Work out the finished part from the listing and answer in its coordinate system (mm). Face numbers are marked on the shaded views. A direction names the side the tool comes from. Coordinates: 2 decimals unless noted, no trailing zeros. Order: outer loops, then holes, each group sorted by start corner. A loop starts at its lowest first (then second) coordinate and runs counter-clockwise, first axis right, second up. Notation, with made-up numbers: M 29.25,-4.75 L 51.25,-4.75 A23 ccw 51.25,15.25 Z; hole C 75,0.5 d8. An arc over 180 degrees is marked long. Use a Markdown table: item, result.
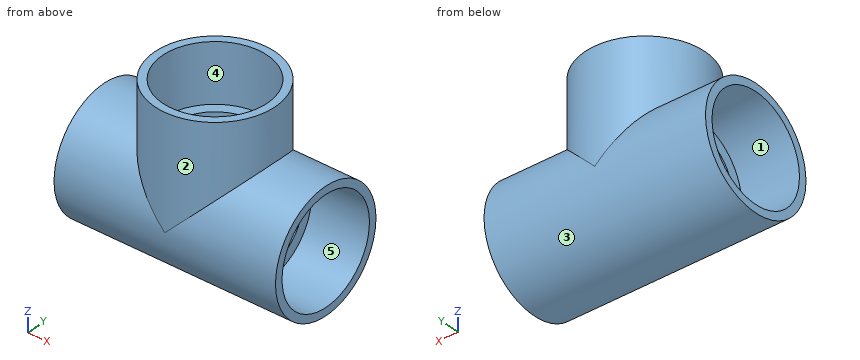
Autodesk Inventor part; units mm, degrees
ref_plane "YZ Plane" through (0, 0, 0) normal (1, 0, 0) x (0, 1, 0)
ref_plane "XZ Plane" through (0, 0, 0) normal (0, 1, 0) x (-1, 0, 0)
ref_plane "XY Plane" through (0, 0, 0) normal (0, 0, 1) x (1, 0, 0)
sketch "Sketch1" plane through (0, 0, 0) normal (0, 1, 0) x (-1, 0, 0)
  line L0 (0, 0) -> (-234, 0)
  line L1 (-234, 0) -> (-234, 63.2)
  line L2 (-234, 63.2) -> (0, 63.2)
  line L3 (0, 63.2) -> (0, 0)
  dimension "d0" = 234
  dimension "d2" = 126.4
revolve "Revolution1" add sketch "Sketch1" angle 360 about axis through (0, 0, 0) along (1, 0, 0)
sketch "Sketch3" plane through (0, 0, 0) normal (0, 1, 0) x (-1, 0, 0)
  line L0 (-180.2, 117) -> (-53.8, 117)
  line L1 (0, -63.2) -> (0, 63.2)
  line L2 (-234, -63.2) -> (-234, 63.2)
  line L3 (0, 0) -> (-234, 0)
  line L4 (-117, 117) -> (-117, 0)
  line L5 (-62, 117) -> (-62, 56)
  line L6 (-62, 56) -> (-73, 56)
  line L7 (-73, 56) -> (-73, 0)
  dimension "d5" = 110
  dimension "d6" = 88
  dimension "d8" = 61
sketch "Sketch2" plane through (0, 0, 0) normal (0, 1, 0) x (-1, 0, 0)
  line L0 (0, 0) -> (-234, 0)
  line L1 (-117, 0) -> (-117, 117)
  line L2 (-117, 117) -> (-53.8, 117)
  line L3 (-53.8, 117) -> (-53.8, 0)
  line L4 (0, -63.2) -> (0, 63.2)
  line L5 (-234, -63.2) -> (-234, 63.2)
  point P0 (-15, 117)
  point P1 (-117, 9)
  dimension "d3" = 126.4
  dimension "d4" = 117
revolve "Revolution2" add sketch "Sketch2" angle 360 about axis through (117, 0, 0) along (0, 0, 1)
revolve "Revolution3" cut sketch "Sketch3" angle 360 about axis through (117, 0, 117) along (0, 0, -1)
sketch "Sketch4" plane through (0, 0, 0) normal (0, 1, 0) x (-1, 0, 0)
  line L0 (0, -63.2) -> (0, 63.2)
  line L1 (-234, -63.2) -> (-234, 63.2)
  line L2 (0, 0) -> (-234, 0)
  line L3 (0, 55) -> (-61, 55)
  line L4 (-61, 55) -> (-61, 44)
  line L5 (-61, 44) -> (-173, 44)
  line L6 (-173, 44) -> (-173, 55)
  line L7 (-173, 55) -> (-234, 55)
  dimension "d9" = 110
  dimension "d10" = 110
  dimension "d11" = 88
  dimension "d12" = 61
  dimension "d14" = 61
revolve "Revolution4" cut sketch "Sketch4" angle 360 about axis through (0, 0, 0) along (1, 0, 0)
equation "\"d0\" = 2 * z1 + 2 * t1"
equation "\"d2\" = d1 + 2 * h1"
equation "\"d5\" = d1"
equation "\"d6\" = 0.8 * d1"
equation "\"d8\" = t1"
equation "\"d9\" = d1"
equation "\"d10\" = d1"
equation "\"d11\" = 0.8 * d1"
equation "\"d12\" = t1"
equation "\"d14\" = t1"
equation "\"d3\" = d1 + 2 * h1"
equation "\"d4\" = z1 + t1"
equation "\"d1\" = 110"
equation "\"z1\" = 56"
equation "\"t1\" = 61"
equation "\"h1\" = 8.2"
properties part number "DIN 8063 Тройник, тип T 110" material "ПВХ, непластифицированный"
1. Section D-D on x = 211.5 is taken. Determine the outline of the cut face in (y, z), then the cut area to 3 significant figures.
Answers below:
| item | result |
|---|---|
| outline | C 0,0 d126.4; hole C 0,0 d110 |
| area | 3,040 mm² |
2. Find the intervals of material crossed by probe 1 along Y at (x, z) = (117, 33); probe 2 along Y at (x, z) = (35.5, 0), in increasing order.
Answers below:
| item | result |
|---|---|
| probe 1 | -63.2 to -44, 44 to 63.2 |
| probe 2 | -63.2 to -55, 55 to 63.2 |
3. Section B-B on x = 117 is taken. Determine the outline of the cut face in (y, z), then the cut area to 3 significant figures.
Answers below:
| item | result |
|---|---|
| outline | M -63.2,0 A63.2 ccw 63.2,0 L 63.2,117 L 55,117 L 55,56 L 44,56 L 44,0 A44 cw -44,0 L -44,56 L -55,56 L -55,117 L -63.2,117 Z |
| area | 6,380 mm² |
4. Section C-C on z = 103.5 is taken. Determine the outline of the cut face in (x, y), then the cut area to 3 significant figures.
Answers below:
| item | result |
|---|---|
| outline | C 117,0 d126.4; hole C 117,0 d110 |
| area | 3,040 mm² |
5. For a pull along Y with two mould halves and no side action, classify the marked faces 1 and 2 as +Y half, -Y half, draft (parallel to the pull), parting line (faces both ways), or undercut.
Answers below:
| item | result |
|---|---|
| face 1 | undercut |
| face 2 | parting line |
6. Flat-ended cylindrical pins translate along their axes: P1, Ø10, axis at x = 87, z = 53.5, coming from the -Y side; P2, Ø1, axis at x = 143.5, y = 3.5, coming from the -Z side; P3, Ø10, axis at x = 45.5, y = -34, coming from the -Z side; P4, Ø2, axis at y = 39.5, z = 50.5, coming from the -X side. Find the tip coordinate at first contact, or state that the pin passes through.
Answers below:
| item | result |
|---|---|
| P1 | y = -58.05 |
| P2 | z = -63.13 |
| P3 | z = -56.15 |
| P4 | x = 0 |
7. For the marked faces 3, 4 and 5, determine the directions among +Z, -Z, +X, -X, +Y, -Y from which every point of the face is accessible in a straight line to the end or side of a thin tool.
Answers below:
| item | result |
|---|---|
| face 3 | none |
| face 4 | +Z |
| face 5 | +X |
8. Section A-A on y = 0 is taken. Determine the outline of the cut face in (x, z).
Answers below:
| item | result |
|---|---|
| outline | M 0,-63.2 L 234,-63.2 L 234,-55 L 173,-55 L 173,-44 L 61,-44 L 61,-55 L 0,-55 Z; M 0,55 L 61,55 L 61,44 L 73,44 L 73,56 L 62,56 L 62,117 L 53.8,117 L 53.8,63.2 L 0,63.2 Z; M 161,44 L 173,44 L 173,55 L 234,55 L 234,63.2 L 180.2,63.2 L 180.2,117 L 172,117 L 172,56 L 161,56 Z |
